Job drawing, mm, ordinate dimensions from the low corner. One solid piece. Round coordinates to 2 decimals unless told otherwise and drop trailing zeros. Loops run counter-clockwise (first coordinate to the right, second up) from the corner with the lowest first, then second, coordinate; pieces in that order, holes last. Notation, with made-up numbers: M -18,40.5 L 27,40.5 A20 cw 27,78.5 Z; hole C 12.25,78.5 d8. An arc over 180 degrees is marked long. Use one line per item in the form item = value.
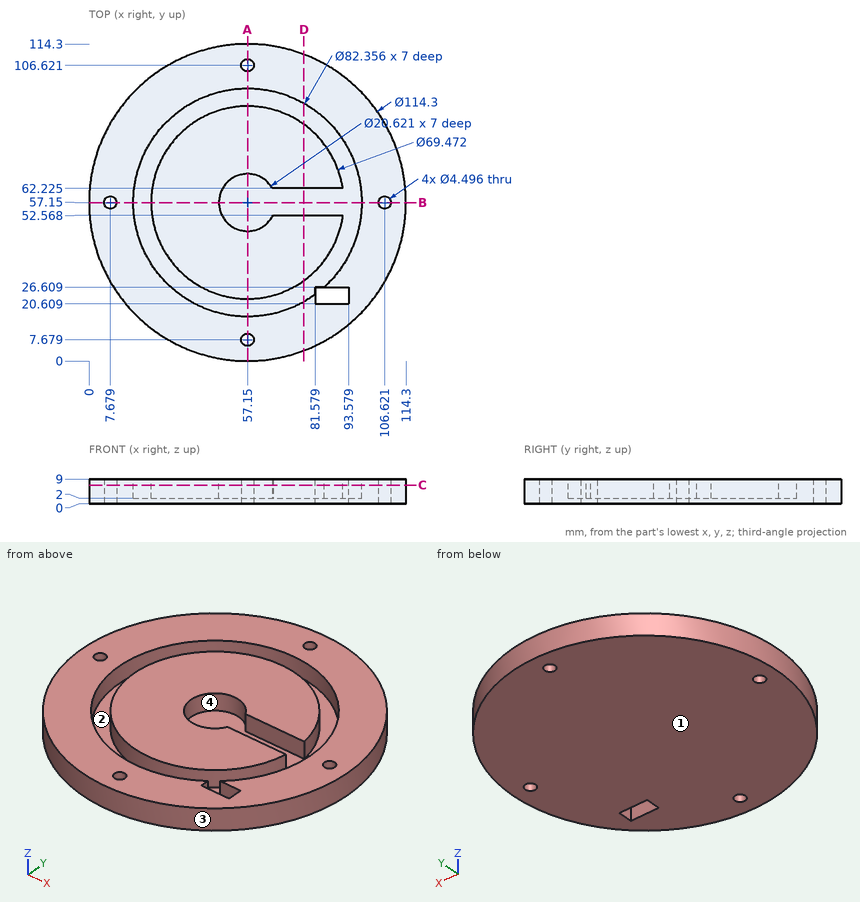
1. Cut at C-C on z = 6.75. State how many separate pieces and enclosed holes the cut face has, and give its area (3 significant figures).
Completed:
separate_pieces = 2
enclosed_holes = 5
area = 8,020 mm2
2. Cut at D-D on x = 77.5. Write the cut outline in (y, z) (1 decimal).
Completed:
outline = M 3.7,0 L 110.6,0 L 110.6,9 L 92.9,9 L 92.9,2 L 85.3,2 L 85.3,9 L 62.2,9 L 62.2,2 L 52.6,2 L 52.6,9 L 29,9 L 29,2 L 21.4,2 L 21.4,9 L 3.7,9 Z
3. Pull direction Y, two halves, no side cores. Call the marked faces 1, 2, 3 and 4: +Y half, -Y half, draft (parallel to the pull), parting line (faces both ways), or undercut.
Completed:
face_1 = draft
face_2 = undercut
face_3 = parting line
face_4 = undercut
4. Probe line 1 along Y through (x, z) = (57.15, 4.75); line 2 along Y through (x, z) = (48.5, 4) (1 decimal); line 3 along X through (y, z) = (82.5, 4). List the from-to ranges inside material, lowest first. Write a range as from..to.
Completed:
line_1 = 0..5.43, 9.93..15.97, 22.41..46.84, 67.46..91.89, 98.33..104.37, 108.87..114.3
line_2 = 0.7..16.9, 23.5..51.5, 62.8..90.8, 97.4..113.6
line_3 = 5.93..24.7, 33.4..80.9, 89.6..108.37
5. Drop flat-ended pins along their axis: P1, Ø3, axis at x = 61, z = 1.5, coming from the +Y side; P2, Ø3.5, axis at x = 73.5, z = 6.5, coming from the +Y side; P3, Ø4.5, axis at x = 85.5, z = 2.5, coming from the -Y side. Give the stop position or say it passes through.
Completed:
P1 = 114.25
P2 = 112.4
P3 = 6.31
6. Cut at A-A on x = 57.15. Write the cut outline in (y, z).
Completed:
outline = M 0,0 L 5.43,0 L 5.43,9 L 0,9 Z; M 9.93,0 L 104.37,0 L 104.37,9 L 98.33,9 L 98.33,2 L 91.89,2 L 91.89,9 L 67.46,9 L 67.46,2 L 46.84,2 L 46.84,9 L 22.41,9 L 22.41,2 L 15.97,2 L 15.97,9 L 9.93,9 Z; M 108.87,0 L 114.3,0 L 114.3,9 L 108.87,9 Z
7. Cut at B-B on y = 57.15. Write the cut outline in (x, z).
Completed:
outline = M 0,0 L 5.43,0 L 5.43,9 L 0,9 Z; M 9.93,0 L 104.37,0 L 104.37,9 L 98.33,9 L 98.33,2 L 46.84,2 L 46.84,9 L 22.41,9 L 22.41,2 L 15.97,2 L 15.97,9 L 9.93,9 Z; M 108.87,0 L 114.3,0 L 114.3,9 L 108.87,9 Z
